The listing builds one solid part. Answer for the finished solid, in the listing's coordinates (mm). A direction names the side the tool comes from. Round coordinates to 2 decimals unless told otherwise and drop trailing zeros. Write each loop counter-clockwise with the first axis right and the second up, starting at its lowest first coordinate (ties: lowest second). Pieces come first, ordered by that corner, then holes. Notation, with made-up numbers: M -4,38 L 25,38 A21 ccw 25,62 Z; hole C -10.75,-30 d4. An arc over 180 degrees is marked long. Put each result on its own line as item: value. Start each with the question number.
```python
from build123d import *

# Parameters (mm, degrees)
F0_W     = 24.9
F0_H     = 17.9
F0_W_2   = 17
F0_H_2   = 1.6
F0_H_3   = 1.9
F1_DEPTH = 4.3
F2_DEPTH = 2.7
F3_DEPTH = 1.6
F4_DEPTH = 1.4


with BuildPart() as f1:
    # F0 (on Top) → F1 (new body)
    with BuildSketch(Plane.XY):
        Polygon((14, -12.731579), (14, 14.368421), (-14.1, 14.368421), (-14.1, -12.731579), (-8.5, -12.731579), (-8.5, -11.131579), (-12.5, -11.131579), (-12.5, -5.131579), (-12.5, 12.768421), (12.4, 12.768421), (12.4, -5.131579), (12.4, -11.131579), (8.5, -11.131579), (8.5, -12.731579), align=None)
        with Locations((-0.05, 3.818421)):
            Rectangle(F0_W, F0_H)
        Polygon((-8.5, -11.131579), (8.5, -11.131579), (12.4, -11.131579), (12.4, -5.131579), (-12.5, -5.131579), (-12.5, -11.131579), align=None)
        with Locations((0, -11.931579)):
            Rectangle(F0_W_2, F0_H_2)
        with Locations((0, -13.681579)):
            Rectangle(F0_W_2, F0_H_3)
    extrude(amount=-F1_DEPTH)

    # F0 (on Top) → F2 (cut)
    with BuildSketch(Plane.XY):
        Polygon((-8.5, -11.131579), (8.5, -11.131579), (12.4, -11.131579), (12.4, -5.131579), (-12.5, -5.131579), (-12.5, -11.131579), align=None)
    extrude(amount=-F2_DEPTH, mode=Mode.SUBTRACT)

    # F0 (on Top) → F3 (cut)
    with BuildSketch(Plane.XY):
        with Locations((-0.05, 3.818421)):
            Rectangle(F0_W, F0_H)
    extrude(amount=-F3_DEPTH, mode=Mode.SUBTRACT)

    # F0 (on Top) → F4 (cut)
    with BuildSketch(Plane.XY):
        with Locations((0, -11.931579)):
            Rectangle(F0_W_2, F0_H_2)
        with Locations((0, -13.681579)):
            Rectangle(F0_W_2, F0_H_3)
    extrude(amount=-F4_DEPTH, mode=Mode.SUBTRACT)


solid = f1.part
```
Item 1: Which of the six approach directions +Z, -Z, +X, -X, +Y, -Y give full straight-line access (tool end or side, diameter ignored) to faces 1 (the flat face through (-12.5, -2, -1)), 2 (the flat face through (-8.5, -12, -1)), 3 (the flat face through (-8.5, -14, -3)), 4 (the flat face through (8.5, -14, -3)), 5 (the flat face through (0, -14.632, -3))?
Item 2: Flat-ended cylindrical pins translate along their axes: pin 1 (1.5 mm diameter, centred on y = -14, z = -3.5, fed in from +X); pin 2 (0.5 mm diameter, centred on x = -4.5, z = -1, fed in from -Y); pin 3 (12 mm diameter, centred on x = 1, y = 5.5, fed in from +Z); pin 4 (10 mm diameter, centred on x = -11, y = 2.5, fed in from +Z). Find the tip coordinate at first contact, or state that the pin passes through.
Item 3: Consider line 1 along X through (y, z) = (-9.25, -1.65); line 2 along Y through (x, z) = (-12.25, -2.6); line 3 along Y through (x, z) = (10.75, -1.35). Determine where each line is inside the solid, lowest interval first. Write a range as [from, to].
Item 4: Section A-A (z = -0.4) is taken. Give the vertices of the cut face in (x, y).
Item 5: Section B-B (y = -11.5) is taken. Give the vertices of the cut face in (x, z), and give its area (3 significant figures).
Item 6: Section D-D (z = -3.15) is taken. Give the vertices of the cut face in (x, y).
Item 7: Determine the mould class of faces 6 (the flat face through (-2, 13, 0)), 7 (the flat face through (0, -5.132, -2)), 8 (the flat face through (11, -12.732, -2)) for opening direction Y: released by +Y, released by -Y, zero draft, split by the parting line, or undercut.
Item 8: Section C-C (x = -1) is taken. Give the vertices of the cut face in (y, z).
Output values:
1. face 1: +Z
1. face 2: +Z, -Y
1. face 3: +Z, -Z, -X, -Y
1. face 4: +Z, -Z, +X, -Y
1. face 5: +Z, -Z, +X, -X, -Y
2. pin 1: stops at x = 8.5
2. pin 2: stops at y = 12.77
2. pin 3: stops at z = -1.6
2. pin 4: stops at z = 0
3. line 1: x = [-14.1, -12.5], [12.4, 14]
3. line 2: y = [-12.73, -11.13], [-5.13, 14.37]
3. line 3: y = [-12.73, -11.13], [12.77, 14.37]
4. outline: M -14.1,-12.73 L -8.5,-12.73 L -8.5,-11.13 L -12.5,-11.13 L -12.5,12.77 L 12.4,12.77 L 12.4,-11.13 L 8.5,-11.13 L 8.5,-12.73 L 14,-12.73 L 14,14.37 L -14.1,14.37 Z
5. outline: M -14.1,-4.3 L 14,-4.3 L 14,0 L 8.5,0 L 8.5,-1.4 L -8.5,-1.4 L -8.5,0 L -14.1,0 Z
5. area: 97.0 mm^2
6. outline: M -14.1,-12.73 L -8.5,-12.73 L -8.5,-14.63 L 8.5,-14.63 L 8.5,-12.73 L 14,-12.73 L 14,14.37 L -14.1,14.37 Z
7. face 6: zero draft
7. face 7: undercut
7. face 8: released by -Y
8. outline: M -14.63,-4.3 L 14.37,-4.3 L 14.37,0 L 12.77,0 L 12.77,-1.6 L -5.13,-1.6 L -5.13,-2.7 L -11.13,-2.7 L -11.13,-1.4 L -14.63,-1.4 Z
